CAD build for the part. Positions are in the model's coordinates, mm. A direction names the side the tool comes from. Round coordinates to 2 decimals unless told otherwise and drop trailing zeros. Loops run counter-clockwise (first coordinate to the right, second up) from the corner with the lowest first, then second, coordinate; pieces in that order, holes last. Notation, with made-up numbers: M 25,58.5 L 65,58.5 A28 ccw 65,88.5 Z; hole C 83.5,59 d1. An arc over 180 degrees is marked long. Put each result on its own line as item: value. Start each with the question number.
from build123d import *

# Parameters (mm, degrees)
SKETCH2_R           = 2.2479
BOSS_EXTRUDE2_DEPTH = 12.7
SKETCH3_R           = 6.35
SKETCH3_W           = 12.7
SKETCH3_H           = 9.756200869
SKETCH3_H_2         = 9.756200868
CUT_EXTRUDE1_DEPTH  = 6.35
CUT_EXTRUDE2_DEPTH  = 6.35


with BuildPart() as part:
    # Sketch2 → Boss-Extrude2 (new body)
    with BuildSketch(Plane(origin=(0, 0, 0), x_dir=(1, 0, 0), z_dir=(0, 1, 0))):
        with BuildLine():
            ThreePointArc((5.556434937, 3.073846253), (-6.34894802, 0.115581283), (5.440872802, -3.274049962))
            Line((5.440872802, -3.274049962), (115.093565063, -5.270254505))
            ThreePointArc((115.093565063, -5.270254505), (126.99894802, -2.311989535), (115.209127198, 1.07764171))
            Line((115.209127198, 1.07764171), (5.556434937, 3.073846253))
        make_face()
        with Locations(Location((120.65, -2.196408252, 0), (0, 0, 270))):
            Circle(SKETCH2_R, mode=Mode.SUBTRACT)
        with Locations(Location((0, 0, 0), (0, 0, 270))):
            Circle(SKETCH2_R, mode=Mode.SUBTRACT)
    extrude(amount=BOSS_EXTRUDE2_DEPTH)

    # Sketch3 → Cut-Extrude1 (cut)
    with BuildSketch(Plane.XZ):
        Circle(SKETCH3_R)
        with Locations((120.65, 2.196408252)):
            Circle(SKETCH3_R)
        with Locations((6.35, -1.471899566)):
            Rectangle(SKETCH3_W, SKETCH3_H)
        with Locations((114.3, 3.668307818)):
            Rectangle(SKETCH3_W, SKETCH3_H_2)
    extrude(amount=-CUT_EXTRUDE1_DEPTH, mode=Mode.SUBTRACT)

    # Sketch4 → Cut-Extrude2 (cut)
    with BuildSketch(Plane.XZ):
        Polygon((47.625, 4.042003257), (47.625, -2.307996743), (73.025, -1.845595005), (73.025, 4.504404995), align=None)
    extrude(amount=-CUT_EXTRUDE2_DEPTH, mode=Mode.SUBTRACT)


solid = part.part
(1) Mould opens along X. For faces 6 (the flat face through (3, 6.35, 0)), 7 (the flat face through (47.625, 3, 1)), 8 (the flat face through (107.95, 3, 2)) say: +X half, -X half, draft (parallel to the pull), parting line (faces both ways), or undercut.
(2) Flat gauge pins, fed straight in: pin 1 Ø2 at (x, y) = (23.5, 3) entering from -Z; pin 2 Ø7 at (y, z) = (2.5, 1) entering from -X; pin 3 Ø2 at (x, z) = (55.5, -3) entering from -Y; pin 4 Ø1 at (x, y) = (10.5, 2.5) entering from +Z. Where does each tip first touch, or does it go through?
(3) Cut at D-D on x = 86. List the corners of the cut face in (y, z), and give its area (3 significant figures).
(4) Drill centre lines: line 1 along Z through (x, y) = (120.65, 8.25); line 2 along X through (y, z) = (6.25, 2.5) (3 decimals); line 3 along Z through (x, y) = (0, 8). Where is each one in solid material? Low to high.
(5) Cut at C-C on y = 10.75. List the corners of the cut face in (x, z), and give its area (3 significant figures).
(6) Cut at B-B on y = 2.5. List the corners of the cut face in (x, z) (3 decimals).
(7) Cut at A-A on x = 0. List the corners of the cut face in (y, z).
(8) Tool access for faces 1 (the flat face through (117, 6.35, 2)), 2 (the flat face through (90, 0, 2)), 3 (the flat face through (12.7, 3, 0)), 4 (the flat face through (73.025, 3, 1)), 5 (the cylindrical face through (-6.34, 9.48, -0.35)): list every direction of +Z, -Z, +X, -X, +Y, -Y with a clear straight run to the whole face (end or side of a thin tool).
Taken from the geometry:
1. face 6: draft
1. face 7: undercut
1. face 8: +X half
2. pin 1: z = -2.77
2. pin 2: x = 12.7
2. pin 3: y = 6.35
2. pin 4: through
3. outline: M 0,-1.61 L 12.7,-1.61 L 12.7,4.74 L 0,4.74 Z
3. area: 80.6 mm2
4. line 1: -4.15 to -0.05, 4.44 to 8.55
4. line 2: 12.7 to 47.625, 73.025 to 107.95
4. line 3: -6.35 to -2.25, 2.25 to 6.35
5. outline: M 5.44,3.27 A6.35 ccw long 5.56,-3.07 L 115.21,-1.08 A6.35 ccw long 115.09,5.27 Z; hole C 0,0 d4.5; hole C 120.65,2.2 d4.5
5. area: 911 mm2
6. outline: M 12.7,-2.944 L 47.625,-2.308 L 47.625,4.042 L 12.7,3.406 Z; M 73.025,-1.846 L 107.95,-1.21 L 107.95,5.14 L 73.025,4.504 Z
7. outline: M 6.35,-6.35 L 12.7,-6.35 L 12.7,-2.25 L 6.35,-2.25 Z; M 6.35,2.25 L 12.7,2.25 L 12.7,6.35 L 6.35,6.35 Z
8. face 1: +Z, -Z, +X, -Y
8. face 2: +Z, -Z, +X, -X, -Y
8. face 3: +Z, -Z, -X, -Y
8. face 4: +Z, -Z, -Y
8. face 5: +Y, -Y
